Could you check a few things on this model? Use its own coordinates, in mm. Face numbers are marked on the shaded views. A direction names the side the tool comes from. Give positions to 0.01 mm unless a question says otherwise; leave off trailing zeros. Loops run counter-clockwise (first coordinate to the right, second up) from the corner with the lowest first, then second, coordinate; pieces in that order, holes last. Notation, with made-up numbers: M 61.25,4 L 82.25,4 A11 ccw 82.25,14 Z; hole C -24.5,24 d1. An arc over 180 degrees is marked long. Answer in a Markdown table with one row per item. Add a question column.
1. Which directions (+Z, -Z, +X, -X, +Y, -Y) give clear straight access to the entire face, cutting with the end or side of a thin tool? Please do the marked faces 4, 5 and 6.
2. If we section it at D-D on x = 0: List the corners of the cut face in (y, z) for me, then the cut area to 3 significant figures.
3. If we section it at A-A on z = 10: List the corners of the cut face in (x, y) for me.
4. I'm going to push flat-ended pins straight in: pin 1 Ø9.5 at (y, z) = (17.03, 10) entering from -X; pin 2 Ø9 at (x, y) = (-2, -0.5) entering from -Z; pin 3 Ø3 at (y, z) = (-4, 9.5) entering from +X. Where does each tip first touch, or does it pass through?
5. I need wall thicknesses on line 1 along X through (y, z) = (0, 17.6); line 2 along Y through (x, z) = (-2.5, 8); line 3 along Y through (x, z) = (2.3, 10). Which ranges of each line are inside material? Lowest first, please. Write a range as from..to.
6. If we section it at B-B on y = 12: List the corners of the cut face in (x, z) for me, then the cut area to 3 significant figures.
7. Thinking about a two-plate mould opening in X: for the marked faces 1, 2 and 3, which applies, released by +X, released by -X, zero draft, split by the parting line, or undercut?
8. If we section it at C-C on z = 15.5: List the corners of the cut face in (x, y) for me.
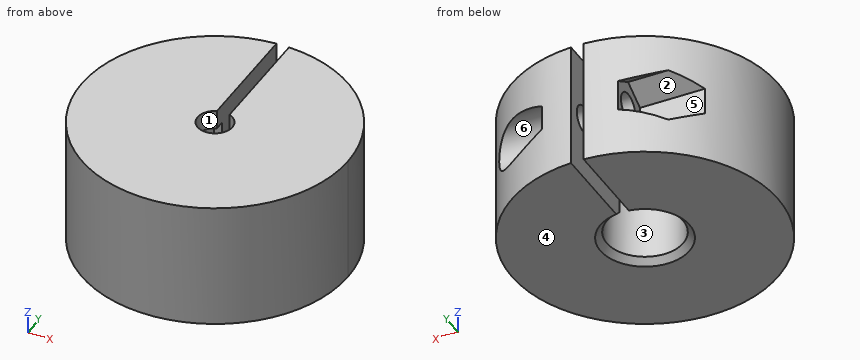
```python
from build123d import *

# Parameters (mm, degrees)
SCHIZZO1_R                    = 21.05
SCHIZZO1_R_2                  = 6.05
ESTRUSIONE_ESTRUSIONE1_DEPTH  = 20
ESTRUSIONE_ESTRUSIONE2_START  = -8
SCHIZZO6_R                    = 6.05
ESTRUSIONE_ESTRUSIONE2_DEPTH  = 8
SCHIZZO8_R                    = 2.75
ESTRUSIONE_ESTRUSIONE3_DEPTH  = 3
SCHIZZO2_W                    = 2
SCHIZZO2_H                    = 24.903468066
TAGLIO_ESTRUSIONE1_DEPTH      = 20
TAGLIO_ESTRUSIONE2_DEPTH      = 37.459635215
TAGLIO_ESTRUSIONE2_DEPTH_BACK = 37.459635215
SCHIZZO3_R                    = 2.2
TAGLIO_ESTRUSIONE3_START      = -5
SCHIZZO4_R                    = 3.7
TAGLIO_ESTRUSIONE3_DEPTH      = 20
TAGLIO_ESTRUSIONE4_START      = -5
TAGLIO_ESTRUSIONE4_DEPTH      = 20
SMUSSO1_SIZE                  = 1


with BuildPart() as part:
    # Schizzo1 → Estrusione-Estrusione1 (new body)
    with BuildSketch(Plane.XY):
        Circle(SCHIZZO1_R)
        Circle(SCHIZZO1_R_2, mode=Mode.SUBTRACT)
    extrude(amount=ESTRUSIONE_ESTRUSIONE1_DEPTH)

    # Schizzo6 → Estrusione-Estrusione2 (add)
    with BuildSketch(Plane.XY.offset(20).offset(ESTRUSIONE_ESTRUSIONE2_START)):
        Circle(SCHIZZO6_R)
        Polygon((2.470277929, 4.03869537), (-2.262473824, 4.158671125), (-4.732751753, 0.119975756), (-2.470277929, -4.03869537), (2.262473824, -4.158671125), (4.732751753, -0.119975756), align=None, mode=Mode.SUBTRACT)
    extrude(amount=ESTRUSIONE_ESTRUSIONE2_DEPTH)

    # Schizzo8 → Estrusione-Estrusione3 (add)
    with BuildSketch(Plane.XY.offset(20)):
        Polygon((-2.262473824, 4.158671125), (-4.732751753, 0.119975756), (-2.470277929, -4.03869537), (2.262473824, -4.158671125), (4.732751753, -0.119975756), (2.470277929, 4.03869537), align=None)
        Circle(SCHIZZO8_R, mode=Mode.SUBTRACT)
    extrude(amount=-ESTRUSIONE_ESTRUSIONE3_DEPTH)

    # Schizzo2 → Taglio-Estrusione1 (cut)
    with BuildSketch(Plane.XY.offset(20)):
        with Locations((0, 13.402032425)):
            Rectangle(SCHIZZO2_W, SCHIZZO2_H)
    extrude(amount=-TAGLIO_ESTRUSIONE1_DEPTH, mode=Mode.SUBTRACT)

    # Schizzo3 → Taglio-Estrusione2 (cut, two sides: drawn at the far end of the back side and taken through both)
    with BuildSketch(Plane.ZY.offset(-1).offset(-TAGLIO_ESTRUSIONE2_DEPTH_BACK)):
        with Locations((10, 17.026233614)):
            Circle(SCHIZZO3_R)
    extrude(amount=TAGLIO_ESTRUSIONE2_DEPTH + TAGLIO_ESTRUSIONE2_DEPTH_BACK, mode=Mode.SUBTRACT)

    # Schizzo4 → Taglio-Estrusione3 (cut)
    with BuildSketch(Plane.ZY.offset(-1).offset(TAGLIO_ESTRUSIONE3_START)):
        with Locations((10, 17.026233614)):
            Circle(SCHIZZO4_R)
    extrude(amount=-TAGLIO_ESTRUSIONE3_DEPTH, mode=Mode.SUBTRACT)

    # Schizzo5 → Taglio-Estrusione4 (cut)
    with BuildSketch(Plane(origin=(-1, 0, 0), x_dir=(0, 0, -1), z_dir=(1, 0, 0)).offset(TAGLIO_ESTRUSIONE4_START)):
        Polygon((-7.863804004, 20.726233614), (-12.136195996, 20.726233614), (-14.272391992, 17.026233614), (-12.136195996, 13.326233614), (-7.863804004, 13.326233614), (-5.727608008, 17.026233614), align=None)
    extrude(amount=-TAGLIO_ESTRUSIONE4_DEPTH, mode=Mode.SUBTRACT)

    # Smusso1
    smusso1_edges = [part.edges().sort_by_distance(p)[0] for p in [
        (0, -6.05, 0),
    ]]
    chamfer(smusso1_edges, length=SMUSSO1_SIZE)


solid = part.part
```
Results:
| question | item | result |
|---|---|---|
| 1 | face 4 | -Z, +X, -X, +Y, -Y |
| 1 | face 5 | -X, +Y |
| 1 | face 6 | +X |
| 2 | outline | M -21.05,0 L -7.05,0 L -6.05,1 L -6.05,12 L -4.1,12 L -4.1,17 L -2.75,17 L -2.75,20 L -21.05,20 Z |
| 2 | area | 319 mm2 |
| 3 | outline | M -16.29,13.33 A21.05 ccw long 16.29,13.33 L 6,13.33 L 6,14.83 L 1,14.83 L 1,5.97 A6.05 cw long -1,5.97 L -1,14.83 L -6,14.83 L -6,13.33 Z; M -6,19.23 L -1,19.23 L -1,21.03 A21.05 ccw -6,20.18 Z; M 1,19.23 L 6,19.23 L 6,20.18 A21.05 ccw 1,21.03 Z |
| 4 | pin 1 | x = -17.1 |
| 4 | pin 2 | z = 0.49 |
| 4 | pin 3 | x = 20.9 |
| 5 | line 1 | -21.05..-2.75, 2.75..21.05 |
| 5 | line 2 | -20.9..-5.51, 5.51..16.11, 17.94..20.9 |
| 5 | line 3 | -20.92..-5.6, 5.6..14.83, 19.23..20.92 |
| 6 | outline | M -17.29,0 L -1,0 L -1,20 L -17.29,20 Z; M 1,0 L 17.29,0 L 17.29,20 L 1,20 Z |
| 6 | area | 652 mm2 |
| 7 | face 1 | undercut |
| 7 | face 2 | zero draft |
| 7 | face 3 | undercut |
| 8 | outline | M -4.73,0.12 L -2.26,4.16 L -1,4.13 L -1,21.03 A21.05 ccw long 1,21.03 L 1,4.08 L 2.47,4.04 L 4.73,-0.12 L 2.26,-4.16 L -2.47,-4.04 Z |
